```python
from build123d import *

# Parameters (mm, degrees)
SKETCH1_W                      = 89
SKETCH1_H                      = 104
BOSS_EXTRUDE1_DEPTH            = 40
SKETCH2_W                      = 83
SKETCH2_H                      = 98
CUT_EXTRUDE1_DEPTH             = 41
F_14_0_14_DIAMETER_HOLE1_D     = 14
F_14_0_14_DIAMETER_HOLE1_DEPTH = 89
F_14_0_14_DIAMETER_HOLE2_D     = 14
F_14_0_14_DIAMETER_HOLE2_DEPTH = 6
FILLET1_R                      = 6
FILLET2_R                      = 12


with BuildPart() as part:
    # Sketch1 → Boss-Extrude1 (new body)
    with BuildSketch(Plane.XY):
        with Locations((44.5, 52)):
            Rectangle(SKETCH1_W, SKETCH1_H)
    extrude(amount=-BOSS_EXTRUDE1_DEPTH)

    # Sketch2 → Cut-Extrude1 (cut, through all)
    with BuildSketch(Plane(origin=(0, 0, -40), x_dir=(-1, 0, 0), z_dir=(0, 0, -1))):
        with Locations((-47.5, 49)):
            Rectangle(SKETCH2_W, SKETCH2_H)
    extrude(amount=-CUT_EXTRUDE1_DEPTH, mode=Mode.SUBTRACT)

    # Ø14.0 (14) Diameter Hole1
    with Locations(Plane.ZY):
        with Locations((-20, 68), (-20, 20)):
            Hole(F_14_0_14_DIAMETER_HOLE1_D / 2, depth=F_14_0_14_DIAMETER_HOLE1_DEPTH)

    # Ø14.0 (14) Diameter Hole2
    with Locations(Plane(origin=(0, 98, 0), x_dir=(-1, 0, 0), z_dir=(0, -1, 0))):
        with Locations((-69, 20), (-21, 20)):
            Hole(F_14_0_14_DIAMETER_HOLE2_D / 2, depth=F_14_0_14_DIAMETER_HOLE2_DEPTH)

    # Fillet1
    fillet1_edges = [part.edges().sort_by_distance(p)[0] for p in [
        (6, 98, -20),
    ]]
    fillet(fillet1_edges, radius=FILLET1_R)

    # Fillet2
    fillet2_edges = [part.edges().sort_by_distance(p)[0] for p in [
        (0, 104, -20),
    ]]
    fillet(fillet2_edges, radius=FILLET2_R)


solid = part.part
```
Here's how the part is built. I have some questions about the finished solid (model axes, mm). A direction names the side the tool comes from. Round coordinates to 2 decimals unless told otherwise and drop trailing zeros. Loops run counter-clockwise (first coordinate to the right, second up) from the corner with the lowest first, then second, coordinate; pieces in that order, holes last.
1. Suppose I cut it at D-D, the plane z = -2.5. Please give me the cut outline in (x, y), and give its area (3 significant figures).
Answers:
outline: (0, 0) - (6, 0) - (6, 92) arc R6 cw to (12, 98) - (89, 98) - (89, 104) - (12, 104) arc R12 ccw to (0, 92) - close
area: 1,100 mm2
2. For faces 1 (the face through (89, 101, -20)), 2 (the face through (51, 98, -20)), which set-ups out of +Z, -Z, +X, -X, +Y, -Y let a thin tool reach every point of the face, with its end or its side?
Answers:
face 1: +Z, -Z, +X, +Y, -Y
face 2: +Z, -Z, +X, -Y
3. Will these pins go through, and if not, where does the flat tip stop? pin 1 (18 mm diameter, centred on y = 20, z = -20, fed in from +X); pin 2 (2 mm diameter, centred on x = 46, z = -35, fed in from -Y).
Answers:
pin 1: stops at x = 6
pin 2: stops at y = 98
4. Suppose I cut it at A-A, the plane x = 69. Please give me the cut outline in (y, z).
Answers:
outline: (98, -40) - (104, -40) - (104, -27) - (98, -27) - close; (98, -13) - (104, -13) - (104, 0) - (98, 0) - close
5. Suppose I cut it at C-C, the plane y = 20. Please give me the cut outline in (x, z).
Answers:
outline: (0, -40) - (6, -40) - (6, -27) - (0, -27) - close; (0, -13) - (6, -13) - (6, 0) - (0, 0) - close
6. Thinking about a two-plate mould opening in X: for faces 3 (the face through (67.483, 101.042, -13.166)), 4 (the face through (3.042, 15.741, -14.445)), 5 (the face through (0, 45, -20)), which applies, released by +X, released by -X, zero draft, split by the parting line, or undercut?
Answers:
face 3: undercut
face 4: zero draft
face 5: released by -X
7. Suppose I cut it at B-B, the plane z = -20. Please give me the cut outline in (x, y), and give its area (3 significant figures).
Answers:
outline: (0, 0) - (6, 0) - (6, 13) - (0, 13) - close; (0, 27) - (6, 27) - (6, 61) - (0, 61) - close; (0, 75) - (6, 75) - (6, 92) arc R6 cw to (12, 98) - (14, 98) - (14, 104) - (12, 104) arc R12 ccw to (0, 92) - close; (28, 98) - (62, 98) - (62, 104) - (28, 104) - close; (76, 98) - (89, 98) - (89, 104) - (76, 104) - close
area: 763 mm2
8. If I drill on probe 1 along X at (y, z) = (100.15, -20); probe 2 along X at (y, z) = (99, -20); probe 3 along Z at (x, y) = (69, 102), over which ranges is the centre line in solid material (lowest first)?
Answers:
probe 1: x = 3.19 to 14, 28 to 62, 76 to 89
probe 2: x = 2.25 to 14, 28 to 62, 76 to 89
probe 3: z = -40 to -27, -13 to 0
